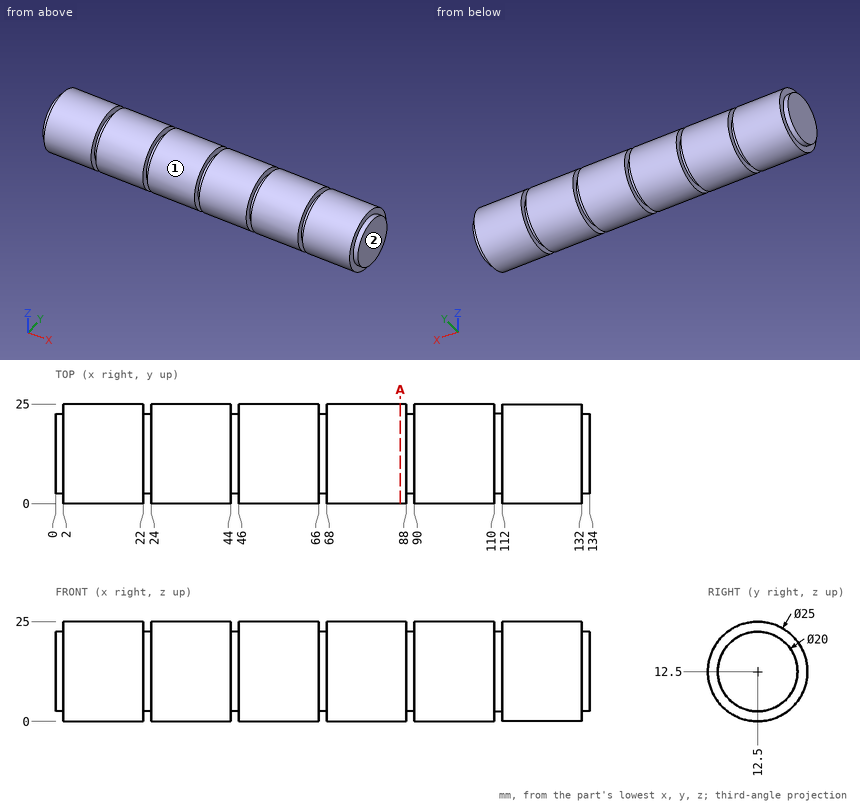
Study the drawing (mm; zero at the part's minimum x, y, z) and answer. Give positions to 0.01 mm unless a question says otherwise; leave off trailing zeros. Order: outer loops, then holes, each group sorted by start corner. A loop starts at its lowest first (then second) coordinate and runs counter-clockwise, first axis right, second up.
1. Section A-A, the plane x = 86.5 is taken. Determine the outline of the cut face in (y, z), and give its area (3 significant figures).
Result sheet:
outline: circle Ø25 at (12.5, 12.5)
area: 491 mm2
2. The mould has two halves that part along Y. Classify the marked faces 1 and 2: released by +Y, released by -Y, zero draft, split by the parting line, or undercut.
Result sheet:
face 1: split by the parting line
face 2: zero draft
3. Each of these flat-tipped pins is pushed along its axis until it touches: P1, Ø7.5, axis at y = 15.5, z = 11, coming from the -X side; P2, Ø4, axis at x = 14, y = 7.5, coming from the -Z side; P3, Ø5, axis at x = 97.5, y = 20.5, coming from the +Z side (3 decimals); P4, Ø2, axis at x = 29, y = 5.5, coming from the -Z side. Where does it stop, or does it pass through?
Result sheet:
P1: stops at x = 0
P2: stops at z = 0.37
P3: stops at z = 23.725
P4: stops at z = 1.53
4. Straight lines are drawn through the part: L1, parallel to X at y = 18.5, z = 1.75; L2, parallel to Y at x = 72.5, z = 12; L3, parallel to Z at x = 28, y = 11. For each, find the intervals that lie inside material, in ascending order.
Result sheet:
L1: x = 2 to 22, 24 to 44, 46 to 66, 68 to 88, 90 to 110, 112 to 132
L2: y = 0.01 to 24.99
L3: z = 0.09 to 24.91
